from build123d import *

# Parameters (mm, degrees)
SKETCH1_R           = 5
SKETCH1_W           = 49.5
SKETCH1_H           = 6
BOSS_EXTRUDE2_DEPTH = 68
SKETCH2_R           = 1.25
BOSS_EXTRUDE3_DEPTH = 4
CUT_EXTRUDE1_START  = -20
SKETCH3_W           = 77.654098362
SKETCH3_H           = 40.574365012
SKETCH3_R           = 5
CUT_EXTRUDE1_DEPTH  = 20


with BuildPart() as part:
    # Sketch1 → Boss-Extrude2 (new body)
    with BuildSketch(Plane(origin=(0, 0, 0), x_dir=(1, 0, 0), z_dir=(0, 1, 0))):
        Circle(SKETCH1_R)
        with Locations((-49.5, 0)):
            Circle(SKETCH1_R)
        with Locations((-24.75, 0)):
            Rectangle(SKETCH1_W, SKETCH1_H)
    extrude(amount=BOSS_EXTRUDE2_DEPTH)

    # Sketch2 → Boss-Extrude3 (add)
    with BuildSketch(Plane(origin=(0, 68, 0), x_dir=(1, 0, 0), z_dir=(0, 1, 0))):
        with Locations(Location((0, 0, 0), (0, 0, 270))):
            Circle(SKETCH2_R)
        with Locations(Location((-49.5, 0, 0), (0, 0, 270))):
            Circle(SKETCH2_R)
    extrude(amount=BOSS_EXTRUDE3_DEPTH)

    # Sketch3 → Cut-Extrude1 (cut)
    with BuildSketch(Plane(origin=(0, 68, 0), x_dir=(1, 0, 0), z_dir=(0, 1, 0)).offset(CUT_EXTRUDE1_START)):
        with Locations((-24.75, -3)):
            Rectangle(SKETCH3_W, SKETCH3_H)
        with Locations(Location((-49.5, 0, 0), (0, 0, 36.869897646))):
            Circle(SKETCH3_R, mode=Mode.SUBTRACT)
        with Locations(Location((0, 0, 0), (0, 0, 143.130102354))):
            Circle(SKETCH3_R, mode=Mode.SUBTRACT)
    extrude(amount=CUT_EXTRUDE1_DEPTH, mode=Mode.SUBTRACT)


solid = part.part
Here's how the part is built. I have some questions about the finished solid (model axes, mm). A direction names the side the tool comes from. Round coordinates to 2 decimals unless told otherwise and drop trailing zeros. Write each loop counter-clockwise with the first axis right and the second up, starting at its lowest first coordinate (ties: lowest second). Pieces come first, ordered by that corner, then holes. Notation, with made-up numbers: (43, 46.25) -> (75, 46.25) arc R16 cw to (75, 67.25) -> close; hole circle Ø5 at (12, -34). An arc over 180 degrees is marked (long way). One line per item, written item: value.
1) Suppose I cut it at C-C on z = 0. List the corners of the cut face in (x, y) for me, plus the area to 3 significant figures.
Filled sheet:
outline: (-54.5, 0) -> (5, 0) -> (5, 68) -> (1.25, 68) -> (1.25, 72) -> (-1.25, 72) -> (-1.25, 68) -> (-5, 68) -> (-5, 48) -> (-44.5, 48) -> (-44.5, 68) -> (-48.25, 68) -> (-48.25, 72) -> (-50.75, 72) -> (-50.75, 68) -> (-54.5, 68) -> close
area: 3,280 mm2
2) Suppose I cut it at D-D on y = 62. List the corners of the cut face in (x, z) for me.
Filled sheet:
outline: circle Ø10 at (-49.5, 0); circle Ø10 at (0, 0)
3) For faces 1 (the face through (-48.26, 69.97, -0.16)), 2 (the face through (-25, 24, 3)), 3 (the face through (-25, 24, -3)), which set-ups out of +Z, -Z, +X, -X, +Y, -Y let a thin tool reach every point of the face, with its end or its side?
Filled sheet:
face 1: +Y
face 2: +Z, +Y, -Y
face 3: -Z, +Y, -Y
4) Suppose I cut it at A-A on z = 4. List the corners of the cut face in (x, y) for me.
Filled sheet:
outline: (-52.5, 0) -> (-46.5, 0) -> (-46.5, 68) -> (-52.5, 68) -> close; (-3, 0) -> (3, 0) -> (3, 68) -> (-3, 68) -> close
5) Suppose I cut it at B-B on x = 0. List the corners of the cut face in (y, z) for me, plus the area to 3 significant figures.
Filled sheet:
outline: (0, -5) -> (68, -5) -> (68, -1.25) -> (72, -1.25) -> (72, 1.25) -> (68, 1.25) -> (68, 5) -> (0, 5) -> close
area: 690 mm2
6) I'm going to push flat-ended pins straight in: pin 1 Ø6 at (x, y) = (-39.5, 15.5) entering from -Z; pin 2 Ø6 at (x, y) = (-5.5, 31) entering from +Z; pin 3 Ø5 at (y, z) = (59.5, -3) entering from +X. Where does each tip first touch, or does it pass through?
Filled sheet:
pin 1: stops at z = -3
pin 2: stops at z = 4.33
pin 3: stops at x = 4.97
7) If I drill on line 1 (Y direction, x = -38.5, z = 1.5); line 2 (Y direction, x = -4.5, z = 0.75); line 3 (X direction, y = 22, z = -0.25), over which ranges is the centre line in solid material (lowest first)? Write a range as [from, to].
Filled sheet:
line 1: y = [0, 48]
line 2: y = [0, 68]
line 3: x = [-54.49, 4.99]
